Input: part model. Units: mm. Frame: model coordinates. A direction names the side the tool comes from. Round coordinates to 2 decimals unless told otherwise and drop trailing zeros. Loops run counter-clockwise (first coordinate to the right, second up) from the corner with the lowest first, then second, coordinate; pieces in that order, holes last. Notation, with made-up numbers: M 89,1 L 140,1 A16 cw 140,32 Z; hole C 83,10 d8. An arc over 180 degrees is marked long. Put each result on its own line as item: value. Start each with the question number.
1) Reachability of faces 5 (the face through (7.006, 3.425, 0.45)), 6 (the face through (38.1, -4, 2)) from +Z, -Z, +X, -X, +Y, -Y: full face, straight path, thin tool, end or side. Return the list, or none.
2) Section A-A on x = 9. Output: boundary loops of the cut face in (y, z) (1 decimal).
3) Section B-B on x = 18. Output: boundary loops of the cut face in (y, z) (1 decimal).
4) Section D-D on y = -6.25. Output: boundary loops of the cut face in (x, z), plus the area to 3 significant figures.
5) Pin query (flat end, axial travel): pin 1 (1.5 mm diameter, centred on x = 16, z = 4.5, fed in from +Y); pin 2 (4 mm diameter, centred on y = 0, z = 0, fed in from -X); pin 3 (5 mm diameter, centred on x = 25, y = 6, fed in from +Z). Return the tip coordinate at first contact, or that it passes through.
6) Section C-C on x = 29. Output: boundary loops of the cut face in (y, z) (1 decimal).
7) Line query: probe 1 along Y at (x, z) = (6.25, 0); probe 2 along Y at (x, z) = (30, 0); probe 3 along Z at (x, y) = (36.5, -5.5). Output: solid intervals per line, ascending.
8) Draft query along Z for faces 1 (the face through (31.12, 0.81, 2.58)), 2 (the face through (19.32, 7.75, 1.72)), 3 (the face through (24.06, 0.14, -0.45)), 4 (the face through (0, 3.4, 3.4)). Return one class per face: +Z half, -Z half, draft (parallel to the pull), parting line (faces both ways), or undercut.
from build123d import *

# Parameters (mm, degrees)
SKETCH1_W                         = 38.1
SKETCH1_H                         = 7.9375
F_1_4_28_TAPPED_HOLE1_D           = 5.4102
F_1_4_28_TAPPED_HOLE1_DEPTH       = 12.7
F_1_4_28_TAPPED_HOLE1_CSINK_D     = 7.62
F_1_4_28_TAPPED_HOLE1_CSINK_ANGLE = 90
F_1_4_28_TAPPED_HOLE1_TIP         = 1.625388061
F_7_16_28_TAPPED_HOLE_D           = 6.9088
F_7_16_28_TAPPED_HOLE_DEPTH       = 12.7
F_7_16_28_TAPPED_HOLE_CSINK_D     = 9.2075
F_7_16_28_TAPPED_HOLE_CSINK_ANGLE = 90
F_7_16_28_TAPPED_HOLE_TIP         = 2.075612922


with BuildPart() as part:
    # Sketch1 → Revolve1 (revolve)
    with BuildSketch(Plane.XY, mode=Mode.PRIVATE) as revolve1_sk:
        with Locations((19.05, 3.96875)):
            Rectangle(SKETCH1_W, SKETCH1_H)
    revolve(revolve1_sk.sketch.rotate(Axis((0, 0, 0), (-1, 0, 0)), 90), axis=Axis((0, 0, 0), (-1, 0, 0)))

    # 1/4-28 Tapped Hole1
    with Locations(Plane(origin=(38.1, 0, 0), x_dir=(0, 0, -1), z_dir=(1, 0, 0))):
        with Locations((0, 0)):
            CounterSinkHole(F_1_4_28_TAPPED_HOLE1_D / 2, F_1_4_28_TAPPED_HOLE1_CSINK_D / 2, depth=F_1_4_28_TAPPED_HOLE1_DEPTH, counter_sink_angle=F_1_4_28_TAPPED_HOLE1_CSINK_ANGLE)
            with Locations((0, 0, -(F_1_4_28_TAPPED_HOLE1_DEPTH + F_1_4_28_TAPPED_HOLE1_TIP / 2))):  # 118° drill point
                Cone(0, F_1_4_28_TAPPED_HOLE1_D / 2, F_1_4_28_TAPPED_HOLE1_TIP, mode=Mode.SUBTRACT)

    # 7/16-28 Tapped Hole
    with Locations(Plane.ZY):
        with Locations((0, 0)):
            CounterSinkHole(F_7_16_28_TAPPED_HOLE_D / 2, F_7_16_28_TAPPED_HOLE_CSINK_D / 2, depth=F_7_16_28_TAPPED_HOLE_DEPTH, counter_sink_angle=F_7_16_28_TAPPED_HOLE_CSINK_ANGLE)
            with Locations((0, 0, -(F_7_16_28_TAPPED_HOLE_DEPTH + F_7_16_28_TAPPED_HOLE_TIP / 2))):  # 118° drill point
                Cone(0, F_7_16_28_TAPPED_HOLE_D / 2, F_7_16_28_TAPPED_HOLE_TIP, mode=Mode.SUBTRACT)


solid = part.part
Geometry results:
1. face 5: -X
1. face 6: +Z, -Z, +X, +Y, -Y
2. outline: C 0,0 d15.9; hole C 0,0 d6.9
3. outline: C 0,0 d15.9
4. outline: M 0,-4.89 L 38.1,-4.89 L 38.1,4.89 L 0,4.89 Z
4. area: 373 mm²
5. pin 1: stops at y = 7
5. pin 2: stops at x = 13.57
5. pin 3: stops at z = 7.12
6. outline: C 0,0 d15.9; hole C 0,0 d5.4
7. probe 1: y = -7.94 to -3.45, 3.45 to 7.94
7. probe 2: y = -7.94 to -2.71, 2.71 to 7.94
7. probe 3: z = -5.72 to 5.72
8. face 1: undercut
8. face 2: parting line
8. face 3: undercut
8. face 4: draft
